Autodesk Inventor part; units mm, degrees
ref_plane "YZ Plane" through (0, 0, 0) normal (1, 0, 0) x (0, 1, 0)
ref_plane "XZ Plane" through (0, 0, 0) normal (0, 1, 0) x (-1, 0, 0)
ref_plane "XY Plane" through (0, 0, 0) normal (0, 0, 1) x (1, 0, 0)
ref_plane "Work Plane1" through (0, 0, 0) normal (0, 0, 1) x (1, 0, 0)
sketch "Sketch1" plane through (0, 0, 0) normal (0, 0, 1) x (1, 0, 0)
  circle A0 centre (12.6053, 80.6735) radius 2.5
  point P0 (0, 0)
  dimension "d0" = 5
extrude "Extrusion1" add sketch "Sketch1" along normal blind 2 and the other way blind 3
sketch "Sketch2" plane through (12.6053, 80.6735, -3) normal (0, 0, -1) x (-1, 0, 0)
  line L0 (-4, -15) -> (4, -15)
  line L1 (4, -15) -> (4, 15)
  line L2 (4, 15) -> (-4, 15)
  line L3 (-4, 15) -> (-4, -15)
  line L4 (-4, -15) -> (4, 15)
  line L5 (-4, -15) -> (27.0483, -15) construction
  circle A0 centre (0, 0) radius 2.5
  point P0 (12.6053, -80.6735)
  dimension "d5" = 8
  dimension "d6" = 30
extrude "Extrusion2" add sketch "Sketch2" along normal blind 2.75
sketch "Sketch5" plane through (12.6053, 80.6735, 2) normal (0, 0, 1) x (1, 0, 0)
  line L0 (4, 15) -> (4, -15)
  line L1 (-4, -15) -> (-4, 15)
  circle A0 centre (0, 0) radius 2.5
  line L2 (-2.25, 1.0897) -> (-2.25, -1.0897)
  line L3 (2.25, 1.0897) -> (2.25, -1.0897)
  circle A1 centre (0, 0) radius 2.5
  point P0 (-12.6053, -80.6735)
  point P1 (2.25, 1.0897)
  point P2 (2.25, -1.0897)
  point P3 (-2.25, -1.0897)
  point P4 (-2.25, 1.0897)
  dimension "d21" = 1.75
  dimension "d22" = 1.75
extrude "Extrusion5" cut sketch "Sketch5" against normal up to surface (5 mm away) contours A0 L3 | L2 A0
fillet "Fillet1" radius 1 4 edges at (12.6053, 83.1735, 2) (12.6053, 78.1735, 2) (10.3553, 80.6735, 2) (14.8553, 80.6735, 2)
sketch "Sketch7" plane through (16.6053, 65.6735, -3) normal (1, 0, 0) x (0, 0, -1)
  line L0 (3.95, 19.8) -> (5.45, 19.8) construction
  line L1 (1.25, 19.15) -> (1.25, 10.85)
  line L2 (0, 30) -> (2.75, 30)
  line L3 (0, 30) -> (0, 0)
  line L4 (0, 0) -> (2.75, 0)
  line L5 (2.75, 30) -> (2.75, 0)
  line L6 (0, 30) -> (2.75, 30)
  line L7 (1.25, 19.15) -> (2.75, 19.15)
  line L8 (2.75, 30) -> (2.75, 0)
  line L9 (1.25, 10.85) -> (2.75, 10.85)
  point P0 (-3, -65.6735)
  point P1 (2.75, 10.85)
  point P2 (2.75, 19.15)
  dimension "d31" = 8.3
  dimension "d52" = 1.5
  dimension "d53" = 10.85
extrude "Extrusion7" cut sketch "Sketch7" against normal blind 5 contours L7 L5 L9 L1
chamfer "Chamfer1" distance 0.7 angle 45 1 edges at (11.6053, 80.6735, -4.25)
sketch "Sketch8" plane through (16.6053, 65.6735, -3) normal (1, 0, 0) x (0, 0, -1)
  line L0 (0, 30) -> (2.75, 30)
  line L1 (0, 30) -> (0, 0)
  line L2 (0, 0) -> (2.75, 0)
  line L3 (0, 0) -> (2.75, 0)
  line L4 (0, 30) -> (2.75, 30)
  line L5 (0.8, 0) -> (0.8, 30)
  line L6 (0, 30) -> (0, 0)
  line L7 (1.8, 0) -> (1.8, 30)
  line L8 (0.8, 6) -> (1.8, 6)
  line L9 (0.8, 24) -> (1.8, 24)
  line L10 (2.75, 30) -> (2.75, 19.15)
  line L11 (2.75, 10.85) -> (1.25, 10.85)
  line L12 (1.25, 10.85) -> (1.25, 19.15)
  line L13 (1.25, 19.15) -> (2.75, 19.15)
  line L14 (2.75, 10.85) -> (2.75, 0)
  point P0 (-3, -65.6735)
  dimension "d38" = 0.8
  dimension "d39" = 1
  dimension "d40" = 6
  dimension "d41" = 6
  dimension "d55" = 0.95
extrude "Extrusion8" cut sketch "Sketch8" against normal up to surface (8 mm away) contours L0 L7 L9 L5 | L5 L8 L7 L2
sketch "Sketch9" plane through (16.6053, 65.6735, -3) normal (1, 0, 0) x (0, 0, -1)
  line L0 (0, 0) -> (0, 30)
  line L1 (0, 30) -> (0, 0)
  ellipse E0 centre (0, 1) end of major axis (0, 2) minor radius 0.5 (0, 2) -> (0, 0) ccw
  ellipse E1 centre (0, 29) end of major axis (0, 30) minor radius 0.5
  point P0 (-3, -65.6735)
  point P1 (0, 28)
  dimension "d48" = 0.5
  dimension "d49" = 0.5
  dimension "d50" = 1
  dimension "d51" = 1
extrude "Extrusion9" add sketch "Sketch9" against normal up to surface (8 mm away) contours E0 L0 | E1 L0 picked at (-0.1666, 28.9882)
properties part number "ON_Off_switch_3DPrint"
Input: part model. Units: mm. Frame: model coordinates. A direction names the side the tool comes from. Give positions to 0.01 mm unless a question says otherwise; leave off trailing zeros. Loops run counter-clockwise (first coordinate to the right, second up) from the corner with the lowest first, then second, coordinate; pieces in that order, holes last. Notation, with made-up numbers: M 81,78 L 123,78 A11 ccw 123,85 Z; hole C 51,-8 d8. An arc over 180 degrees is marked long. Use CSV: the item, a comma, the result in double quotes.
(1) Material intervals for L1, parallel to Z at x = 13, y = 70.75; L2, parallel to Y at x = 14, z = -5.25; L3, parallel to Z at x = 9, y = 75, sorted ascending. Write a range as [from, to].
Outcome:
L1,"z = [-5.75, -4.8], [-3.8, -3]"
L2,"y = [65.67, 76.52], [84.82, 95.67]"
L3,"z = [-5.75, -3]"
(2) Set-up query: faces 1 (the face through (13, 89.674, -4)), 2 (the face through (13, 69, -4.8)), 3 (the face through (14, 76.524, -5)). Return all of +Z, -Z, +X, -X, +Y, -Y with unobstructed straight access to the full face (end or side cutting, diameter ignored); none if empty.
Outcome:
face 1,"+X, -X, +Y"
face 2,"+X, -X, -Y"
face 3,"-Z, +X"
(3) Pull-direction query (Y, two-part tool) for faces 4 (the face through (14, 81, -4.25)), 5 (the face through (16.605, 81, -4)), 6 (the face through (13, 95.674, -5)); classes: pulls with the +Y half, pulls with the -Y half, needs draft (parallel to the pull), parting line crosses it, or undercut.
Outcome:
face 4,"undercut"
face 5,"needs draft"
face 6,"pulls with the +Y half"
(4) Pin query (flat end, axial travel): P1, Ø2.5, axis at x = 10.5, y = 86.5, coming from the +Z side; P2, Ø2.5, axis at y = 80.5, z = -1, coming from the -X side; P3, Ø4.5, axis at x = 15, y = 80.5, coming from the -Z side. Return the tip coordinate at first contact, or that it passes through.
Outcome:
P1,"stops at z = -3"
P2,"stops at x = 10.36"
P3,"stops at z = -4.25"
(5) Section A-A, the plane y = 70. Return loops of the section in (x, z), plus the area to 3 significant figures.
Outcome:
outline,"M 8.61,-5.75 L 16.61,-5.75 L 16.61,-4.8 L 8.61,-4.8 Z; M 8.61,-3.8 L 16.61,-3.8 L 16.61,-3 L 8.61,-3 Z"
area,"14.0 mm²"
(6) Section B-B, the plane z = 0.5. Return loops of the section in (x, y).
Outcome:
outline,"M 10.36,79.58 A2.5 ccw 14.86,79.58 L 14.86,81.76 A2.5 ccw 10.36,81.76 Z"
